Source: three-view drawing plus pictorial views. Frame: mm from the lowest corner of the part. Give positions to 0.01 mm unless a question says otherwise; leave off trailing zeros. Order: outer loops, then holes, each group sorted by start corner. A loop starts at its lowest first (then second) coordinate and runs counter-clockwise, first axis right, second up. Notation, with made-up numbers: M 14.5,-16 L 65.5,-16 A19 ccw 65.5,0 Z; hole C 64.5,-12.75 d10. An arc over 180 degrees is marked long. Use CSV: the item, a comma, the result in double quotes. Start each with the question number.
1. Section query A-A, the plane z = 137. Return the cut outline in (x, y).
2. Pin query (flat end, axial travel): P1, Ø3.5, axis at x = 227.5, z = 147, coming from the +Y side; P2, Ø3, axis at y = 17, z = 26, coming from the +X side; P3, Ø13, axis at x = 31.5, y = 17.5, coming from the +Z side. Return the tip coordinate at first contact, or that it passes through.
3. Line query: line 1 along Z through (x, y) = (227.5, 4.5); line 2 along X through (y, z) = (5, 25); line 3 along X through (y, z) = (8.25, 21). Output: solid intervals per line, ascending. Write a range as [from, to].
4. Section query B-B, the plane x = 184.5. Return the cut outline in (y, z), plus the area to 3 significant figures.
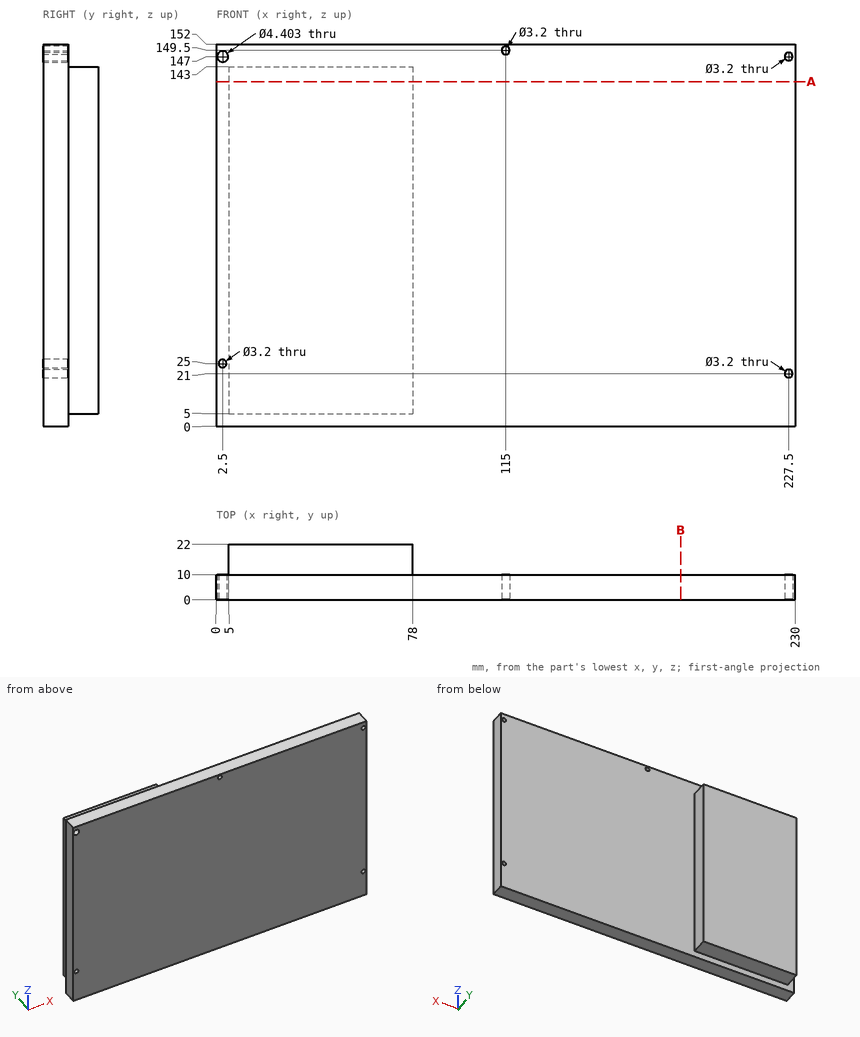
Result set:
1,outline,"M 0,0 L 230,0 L 230,10 L 78,10 L 78,22 L 5,22 L 5,10 L 0,10 Z"
2,P1,"y = 10"
2,P2,"x = 78"
2,P3,"z = 143"
3,line 1,"[0, 19.4], [22.6, 145.4], [148.6, 152]"
3,line 2,"[0, 0.9], [4.1, 230]"
3,line 3,"[0, 225.9], [229.1, 230]"
4,outline,"M 0,0 L 10,0 L 10,152 L 0,152 Z"
4,area,"1,520 mm2"
